The model under review builds one solid part; all positions refer to its coordinate system, in mm. Face numbers are marked on the shaded views. A direction names the side the tool comes from. Coordinates: 2 decimals unless noted, no trailing zeros. Order: outer loops, then holes, each group sorted by start corner. A loop starts at its lowest first (then second) coordinate and runs counter-clockwise, first axis right, second up.
from build123d import *

# Parameters (mm, degrees)
F0_W     = 32.3
F0_H     = 32.3
F0_R     = 1.15
F1_DEPTH = 1.2
F0_R_2   = 7.8
F0_W_2   = 2.5
F0_H_2   = 3.62
F2_DEPTH = 8.14
F3_DEPTH = 11.08
F4_R     = 5.9
F5_DEPTH = 19.5
F6_START = 15.2
F4_R_2   = 7
F6_DEPTH = 4.3


with BuildPart() as f1:
    # F0 (on Top) → F1 (new body)
    with BuildSketch(Plane.XY):
        Rectangle(F0_W, F0_H)
        with Locations((-14.2, -14.2)):
            Circle(F0_R, mode=Mode.SUBTRACT)
        with Locations((14.2, -14.2)):
            Circle(F0_R, mode=Mode.SUBTRACT)
        with BuildLine():
            Line((-8.15, 1.81), (-8.15, 8.15))
            Line((-8.15, 8.15), (-2.15, 8.15))
            Line((-2.15, 8.15), (-2.15, 10))
            ThreePointArc((-2.15, 10), (0, 12.15), (2.15, 10))
            Line((2.15, 10), (2.15, 8.15))
            Line((2.15, 8.15), (8.15, 8.15))
            Line((8.15, 8.15), (8.15, -8.15))
            Line((8.15, -8.15), (2.15, -8.15))
            Line((2.15, -8.15), (2.15, -10))
            ThreePointArc((2.15, -10), (0, -12.15), (-2.15, -10))
            Line((-2.15, -10), (-2.15, -8.15))
            Line((-2.15, -8.15), (-8.15, -8.15))
            Line((-8.15, -8.15), (-8.15, -1.81))
            Line((-8.15, -1.81), (-10.65, -1.81))
            Line((-10.65, -1.81), (-10.65, 1.81))
            Line((-10.65, 1.81), (-8.15, 1.81))
        make_face(mode=Mode.SUBTRACT)
        with Locations((-14.2, 14.2)):
            Circle(F0_R, mode=Mode.SUBTRACT)
        with Locations((14.2, 14.2)):
            Circle(F0_R, mode=Mode.SUBTRACT)
    extrude(amount=F1_DEPTH)

    # F0 (on Top) → F2 (join)
    with BuildSketch(Plane.XY):
        with BuildLine():
            Line((1.095445115, 8.15), (-1.095445115, 8.15))
            ThreePointArc((-1.095445115, 8.15), (0, 7.85), (1.095445115, 8.15))
        make_face()
        with BuildLine():
            ThreePointArc((1.095445115, -8.15), (0, -7.85), (-1.095445115, -8.15))
            Line((-1.095445115, -8.15), (1.095445115, -8.15))
        make_face()
        with BuildLine():
            Line((-1.095445115, -8.15), (-2.15, -8.15))
            Line((-2.15, -8.15), (-2.15, -10))
            ThreePointArc((-2.15, -10), (-1.86784729, -8.9352716302), (-1.095445115, -8.15))
        make_face()
        with BuildLine():
            Line((2.15, -8.15), (1.095445115, -8.15))
            ThreePointArc((1.095445115, -8.15), (1.86784729, -8.9352716302), (2.15, -10))
            Line((2.15, -10), (2.15, -8.15))
        make_face()
        with BuildLine():
            Line((1.095445115, -8.15), (-1.095445115, -8.15))
            ThreePointArc((-1.095445115, -8.15), (-1.86784729, -8.9352716302), (-2.15, -10))
            ThreePointArc((-2.15, -10), (0, -12.15), (2.15, -10))
            ThreePointArc((2.15, -10), (1.86784729, -8.9352716302), (1.095445115, -8.15))
        make_face()
        with BuildLine():
            ThreePointArc((2.15, 10), (1.86784729, 8.9352716302), (1.095445115, 8.15))
            Line((1.095445115, 8.15), (2.15, 8.15))
            Line((2.15, 8.15), (2.15, 10))
        make_face()
        with BuildLine():
            Line((-2.15, 10), (-2.15, 8.15))
            Line((-2.15, 8.15), (-1.095445115, 8.15))
            ThreePointArc((-1.095445115, 8.15), (-1.86784729, 8.9352716302), (-2.15, 10))
        make_face()
        with BuildLine():
            ThreePointArc((-2.15, 10), (-1.86784729, 8.9352716302), (-1.095445115, 8.15))
            Line((-1.095445115, 8.15), (1.095445115, 8.15))
            ThreePointArc((1.095445115, 8.15), (1.86784729, 8.9352716302), (2.15, 10))
            ThreePointArc((2.15, 10), (0, 12.15), (-2.15, 10))
        make_face()
        with BuildLine():
            Line((-2.15, 8.15), (-8.15, 8.15))
            Line((-8.15, 8.15), (-8.15, 1.81))
            Line((-8.15, 1.81), (-8.15, -1.81))
            Line((-8.15, -1.81), (-8.15, -8.15))
            Line((-8.15, -8.15), (-2.15, -8.15))
            Line((-2.15, -8.15), (-1.095445115, -8.15))
            ThreePointArc((-1.095445115, -8.15), (0, -7.85), (1.095445115, -8.15))
            Line((1.095445115, -8.15), (2.15, -8.15))
            Line((2.15, -8.15), (8.15, -8.15))
            Line((8.15, -8.15), (8.15, 8.15))
            Line((8.15, 8.15), (2.15, 8.15))
            Line((2.15, 8.15), (1.095445115, 8.15))
            ThreePointArc((1.095445115, 8.15), (0, 7.85), (-1.095445115, 8.15))
            Line((-1.095445115, 8.15), (-2.15, 8.15))
        make_face()
        Circle(F0_R_2, mode=Mode.SUBTRACT)
        with Locations((-9.4, 0)):
            Rectangle(F0_W_2, F0_H_2)
    extrude(amount=F2_DEPTH)

    # F0 (on Top) → F3 (join)
    with BuildSketch(Plane.XY):
        Circle(F0_R_2)
    extrude(amount=F3_DEPTH)

    # F4 (on Top) → F5 (join)
    with BuildSketch(Plane.XY):
        Circle(F4_R)
    extrude(amount=F5_DEPTH)

    # F4 (on Top) → F6 (join)
    with BuildSketch(Plane.XY.offset(F6_START)):
        Circle(F4_R_2)
        Circle(F4_R, mode=Mode.SUBTRACT)
    extrude(amount=F6_DEPTH)


solid = f1.part
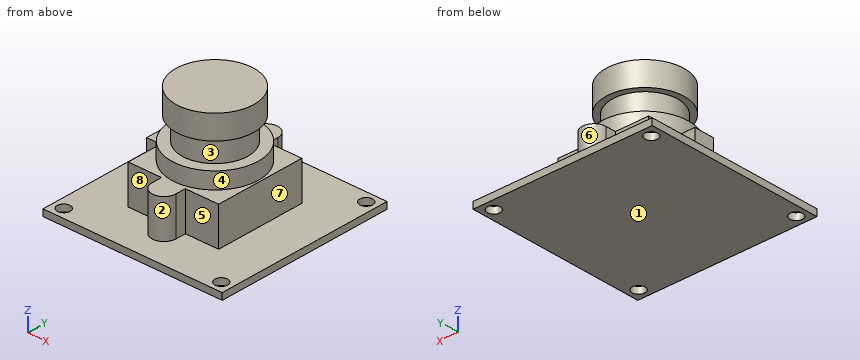
(1) Tool access review of the marked faces 4, 5, 6, 7 and 8: name each direction out of +Z, -Z, +X, -X, +Y, -Y from which nothing blocks a thin tool from reaching the whole face with its end or side.
(2) Wall thickness on line 1 (Y direction, x = -14.2, z = 0.95); line 2 (X direction, y = 4, z = 5.5); line 3 (Z direction, x = 12, y = 11): over which ranges is each line inside the solid? List them lowest first.
(3) Consider section C-C (y = 0). Give the boundary of the cut face in (x, z), then the cut area to 3 significant figures.
(4) Consider section D-D (x = 0). Give the boundary of the cut face in (y, z).
(5) Insertion check: pin 1 Ø3 at (y, z) = (-0.5, 4.5) entering from -X; pin 2 Ø2 at (y, z) = (3.5, 5) entering from +X; pin 3 Ø4 at (x, z) = (-12.5, 8.5) entering from -Y. Each pin has a flat end and moves straight along its axis. Give the tip position at first contact, or say it passes through.
(6) The part is to be moulded in two halves that separate along Z. For the marked faces 1, 2 and 3, say which applies: +Z half, -Z half, draft (parallel to the pull), parting line (faces both ways), or undercut.
(7) Consider section A-A (y = -14.2). Give the boundary of the cut face in (x, z), then the cut area to 3 significant figures.
Findings:
1. face 4: +Z
1. face 5: +Z, +X, -Y
1. face 6: +Z, +Y
1. face 7: +Z, +X, +Y, -Y
1. face 8: +Z, -X, -Y
2. line 1: y = -16.15 to -15.35, -13.05 to 13.05, 15.35 to 16.15
2. line 2: x = -8.15 to 8.15
2. line 3: z = 0 to 1.2
3. outline: (-16.15, 0) - (16.15, 0) - (16.15, 1.2) - (8.15, 1.2) - (8.15, 8.14) - (7.8, 8.14) - (7.8, 11.08) - (5.9, 11.08) - (5.9, 15.2) - (7, 15.2) - (7, 19.5) - (-7, 19.5) - (-7, 15.2) - (-5.9, 15.2) - (-5.9, 11.08) - (-7.8, 11.08) - (-7.8, 8.14) - (-10.65, 8.14) - (-10.65, 1.2) - (-16.15, 1.2) - close
3. area: 324 mm2
4. outline: (-16.15, 0) - (16.15, 0) - (16.15, 1.2) - (12.15, 1.2) - (12.15, 8.14) - (7.8, 8.14) - (7.8, 11.08) - (5.9, 11.08) - (5.9, 15.2) - (7, 15.2) - (7, 19.5) - (-7, 19.5) - (-7, 15.2) - (-5.9, 15.2) - (-5.9, 11.08) - (-7.8, 11.08) - (-7.8, 8.14) - (-12.15, 8.14) - (-12.15, 1.2) - (-16.15, 1.2) - close
5. pin 1: stops at x = -10.65
5. pin 2: stops at x = 8.15
5. pin 3: stops at y = -1.81
6. face 1: -Z half
6. face 2: draft
6. face 3: undercut
7. outline: (-16.15, 0) - (-15.35, 0) - (-15.35, 1.2) - (-16.15, 1.2) - close; (-13.05, 0) - (13.05, 0) - (13.05, 1.2) - (-13.05, 1.2) - close; (15.35, 0) - (16.15, 0) - (16.15, 1.2) - (15.35, 1.2) - close
7. area: 33.2 mm2
